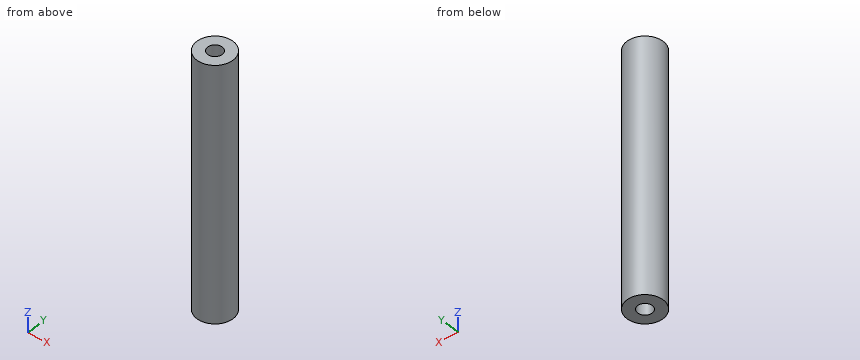
Autodesk Inventor part; units mm, degrees
ref_plane "YZ Plane" through (0, 0, 0) normal (1, 0, 0) x (0, 1, 0)
ref_plane "XZ Plane" through (0, 0, 0) normal (0, 1, 0) x (-1, 0, 0)
ref_plane "XY Plane" through (0, 0, 0) normal (0, 0, 1) x (1, 0, 0)
sketch "Esquisse1" plane through (0, 0, 0) normal (0, 0, 1) x (1, 0, 0)
  circle A0 centre (0, 0) radius 2.5
  dimension "d0" = 5
extrude "Extrusion1" add sketch "Esquisse1" along normal blind 35
sketch "Esquisse2" plane through (0, 0, 35) normal (0, 0, 1) x (1, 0, 0)
  point P0 (0, 0)
  point P1 (0, 0)
sketch "Esquisse3" plane through (0, 0, 0) normal (0, 0, -1) x (-1, 0, 0)
  point P0 (0, 0)
  point P1 (0, 0)
hole "Perçage1" at (0, 0, 0) direction (0, 0, 1) diameter 2 depth 8 tip angle 118
hole "Perçage2" at (0, 0, 35) direction (0, 0, -1) diameter 2 depth 8 tip angle 118
properties part number "elevateur support"
For this review, take the finished solid that the model builds, in its own axes (mm). Give positions to 0.01 mm unless a question says otherwise; leave off trailing zeros. Loops run counter-clockwise (first coordinate to the right, second up) from the corner with the lowest first, then second, coordinate; pieces in that order, holes last. Notation, with made-up numbers: M 28.5,77 L 84.5,77 A7 cw 84.5,82 Z; hole C -32.5,84.5 d8. An arc over 180 degrees is marked long. Put each result on its own line as item: value. Start each with the question number.
(1) Add section D-D, the plane x = 1.9. Write out the cut boundary in (y, z), then the cut area to 3 significant figures.
(2) Add section B-B, the plane z = 13. Write out the cut boundary in (x, y).
(3) Add section C-C, the plane x = -1.4. Write out the cut boundary in (y, z), then the cut area to 3 significant figures.
(4) For pin 1 (1.8 mm diameter, centred on x = 0, y = 0, fed in from +Z), flat-tipped, find the tip position at first contact; note if it passes through.
(5) Add section A-A, the plane z = 7.5. Write out the cut boundary in (x, y).
(6) Wall thickness on L1, parallel to Y at x = 0, z = 5.75; L2, parallel to X at y = -0.1, z = 28; L3, parallel to X at y = 0.1, z = 13: over which ranges is each line inside the solid? List them lowest first.
Result:
1. outline: M -1.62,0 L 1.62,0 L 1.62,35 L -1.62,35 Z
1. area: 114 mm^2
2. outline: C 0,0 d5
3. outline: M -2.07,0 L 2.07,0 L 2.07,35 L -2.07,35 Z
3. area: 145 mm^2
4. pin 1: stops at z = 26.94
5. outline: C 0,0 d5; hole C 0,0 d2
6. L1: y = -2.5 to -1, 1 to 2.5
6. L2: x = -2.5 to -0.99, 0.99 to 2.5
6. L3: x = -2.5 to 2.5
